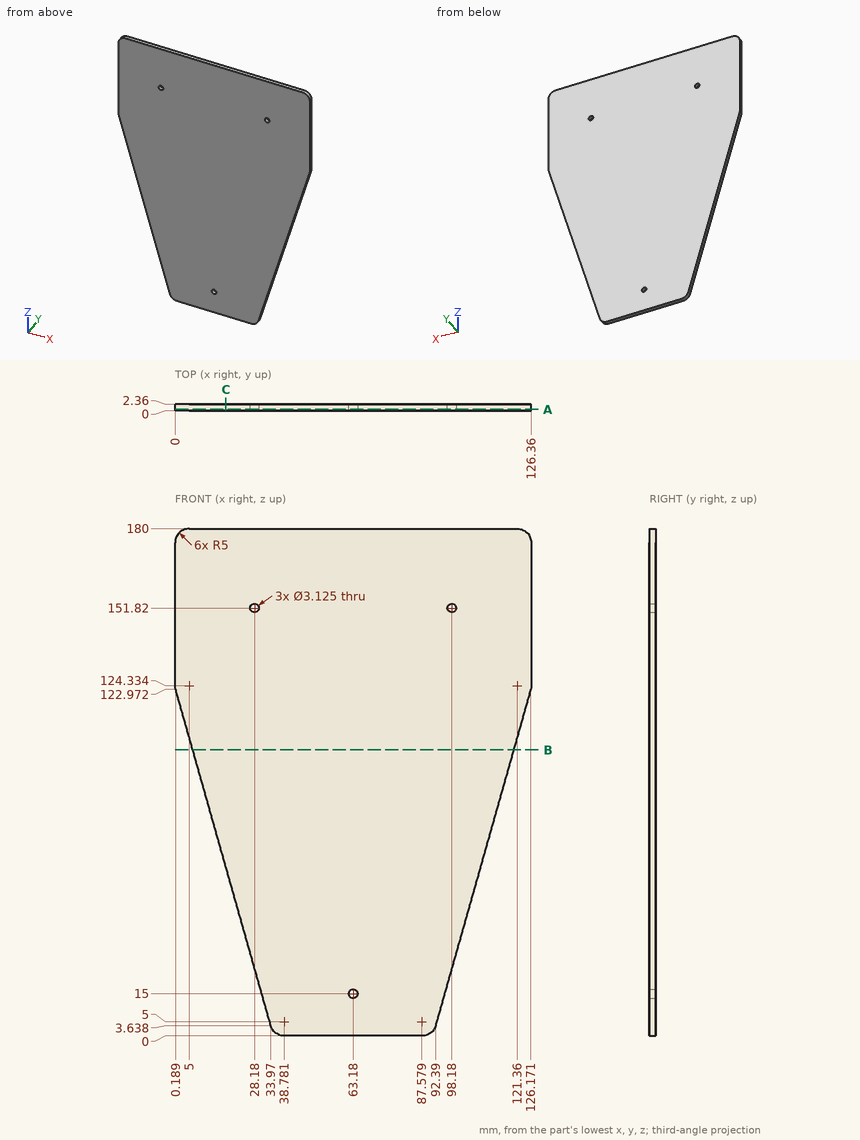
Verification items for this drawing (mm, ordinates from the low corner). Coordinates: 2 decimals unless noted, no trailing zeros. Write each loop counter-clockwise with the first axis right and the second up, starting at its lowest first coordinate (ties: lowest second). Pieces come first, ordered by that corner, then holes. Notation, with made-up numbers: M -20.5,18 L -7.5,18 A21 ccw -7.5,46 Z; hole C 6.25,33.25 d6. An arc over 180 degrees is marked long. One line per item, written item: value. Start each with the question number.
(1) Scan lines: line 1 along X through (y, z) = (0.9, 151.82); line 2 along Z through (x, y) = (63.18, 1.75); line 3 along X through (y, z) = (1.65, 30.5). Record each from-to range of solid material in increasing order. Write a range as [from, to].
(2) Sectioned sample at A-A, the plane y = 0.45. Enter the section's corners in (x, z) (1 decimal).
(3) Sectioned sample at B-B, the plane z = 101.5. Enter the section's corners in (x, y), and give its area (3 significant figures).
(4) Sectioned sample at C-C, the plane x = 18. Enter the section's corners in (y, z), and give its area (3 significant figures).
Filled sheet:
1. line 1: [0, 26.62], [29.74, 96.62], [99.74, 126.36]
1. line 2: [0, 13.44], [16.56, 180]
1. line 3: [26.37, 99.99]
2. outline: M 0,124.3 A5 ccw 0.2,123 L 34,3.6 A5 ccw 38.8,0 L 87.6,0 A5 ccw 92.4,3.6 L 126.2,123 A5 ccw 126.4,124.3 L 126.4,175 A5 ccw 121.4,180 L 5,180 A5 ccw 0,175 Z; hole C 28.2,151.8 d3.1; hole C 63.2,15 d3.1; hole C 98.2,151.8 d3.1
3. outline: M 6.27,0 L 120.09,0 L 120.09,2.36 L 6.27,2.36 Z
3. area: 269 mm²
4. outline: M 0,60.05 L 2.36,60.05 L 2.36,180 L 0,180 Z
4. area: 283 mm²
